Could you check a few things on this drawing? It's one solid part, dimensions in mm from its lowest x, y, z. Give positions to 0.01 mm unless a question says otherwise; leave off trailing zeros. Write each loop counter-clockwise with the first axis right and the second up, starting at its lowest first coordinate (ties: lowest second). Pieces come first, ordered by that corner, then holes. Notation, with made-up numbers: (-33, 74.5) -> (-29, 74.5) arc R15 ccw to (-29, 102.5) -> close; hole circle Ø2 at (-10, 16.5). An arc over 180 degrees is marked (long way). Use CSV: the item, a comma, the result in double quotes. Start each with the question number.
(1) For pin 1 Ø11 at (x, z) = (14.25, 31.75) entering from +Y, with a flat end and sliding along its axis, tell me the tip position at first contact or that it passes through.
(2) Suppose I cut it at A-A on z = 31.75. Give the number of separate pieces and of enclosed holes in the cut face, plus the area to 3 significant figures.
(3) I need wall thicknesses on L1, parallel to X at y = 4.65, z = 29 (1 decimal); L2, parallel to Z at x = 31.75, y = 3.95; L3, parallel to Z at x = 33.5, y = 0.95 (1 decimal). Which ranges of each line are inside material? Lowest first, please. Write a range as [from, to].
(4) Suppose I cut it at C-C on x = 31.75. List the corners of the cut face in (y, z) for me.
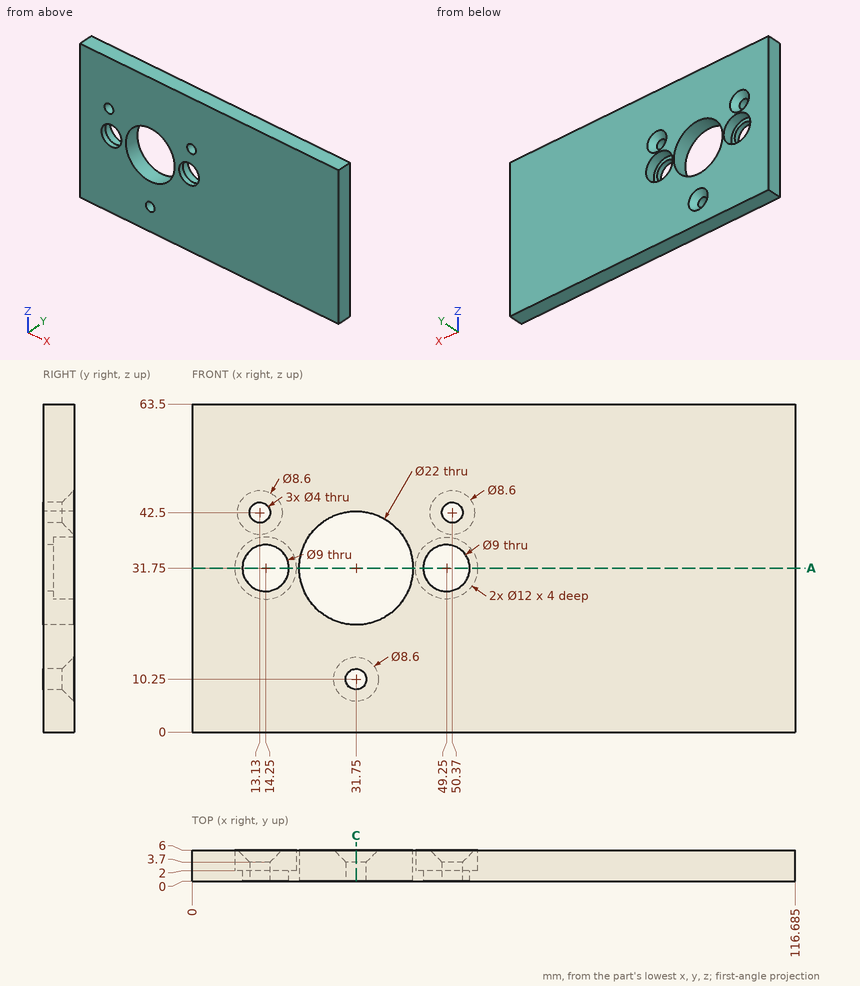
Geometry says:
1,pin 1,"y = 2"
2,separate pieces,"4"
2,enclosed holes,"0"
2,area,"436 mm²"
3,L1,"[0, 8.9], [19.6, 21.1], [42.4, 43.9], [54.6, 116.7]"
3,L2,"[0, 8], [12.5, 20.75], [42.75, 63.5]"
3,L3,"[0, 9.3], [11.2, 20.9], [42.6, 63.5]"
4,outline,"(0, 0) -> (6, 0) -> (6, 5.95) -> (3.7, 8.25) -> (0, 8.25) -> close; (0, 12.25) -> (3.7, 12.25) -> (6, 14.55) -> (6, 20.75) -> (0, 20.75) -> close; (0, 42.75) -> (6, 42.75) -> (6, 63.5) -> (0, 63.5) -> close"
